from build123d import *

# Parameters (mm, degrees)
SKETCH1_W           = 35
SKETCH1_H           = 35
BOSS_EXTRUDE1_DEPTH = 9.6
SKETCH2_R           = 10
SKETCH2_R_2         = 8
CUT_EXTRUDE1_DEPTH  = 7.6
CUT_EXTRUDE2_DEPTH  = 2
CHAMFER1_SIZE       = 2.5
SKETCH4_R           = 1.65
SKETCH4_R_2         = 2.25
CUT_EXTRUDE3_DEPTH  = 26.889380062
SKETCH5_R           = 3
CUT_EXTRUDE4_DEPTH  = 2.5
BOSS_EXTRUDE3_DEPTH = 1.25


with BuildPart() as part:
    # Sketch1 → Boss-Extrude1 (new body)
    with BuildSketch(Plane(origin=(0, 0, 0), x_dir=(1, 0, 0), z_dir=(0, 1, 0))):
        Rectangle(SKETCH1_W, SKETCH1_H)
    extrude(amount=BOSS_EXTRUDE1_DEPTH)

    # Sketch2 → Cut-Extrude1 (cut)
    # profile 1 of 2: a face of its own
    with BuildSketch(Plane(origin=(0, 9.6, 0), x_dir=(1, 0, 0), z_dir=(0, 1, 0))):
        Polygon((16.25, 7), (7, 16.25), (-7, 16.25), (-16.25, 7), (-16.25, -7), (-7, -16.25), (-4, -16.25), (-4, -17.5), (4, -17.5), (4, -16.25), (7, -16.25), (16.25, -7), align=None)
        with Locations(Location((0, 0, 0), (0, 0, 270))):
            Circle(SKETCH2_R, mode=Mode.SUBTRACT)
    # profile 2 of 2: a face of its own
    with BuildSketch(Plane(origin=(0, 9.6, 0), x_dir=(1, 0, 0), z_dir=(0, 1, 0))):
        with Locations(Location((0, 0, 0), (0, 0, 270))):
            Circle(SKETCH2_R_2)
    extrude(amount=-CUT_EXTRUDE1_DEPTH, mode=Mode.SUBTRACT)

    # Sketch3 → Cut-Extrude2 (cut)
    with BuildSketch(Plane(origin=(0, 9.6, 0), x_dir=(1, 0, 0), z_dir=(0, 1, 0))):
        Polygon((11.75, 17.5), (-11.75, 17.5), (-17.5, 11.75), (-17.5, -11.75), (-11.75, -17.5), (11.75, -17.5), (17.5, -11.75), (17.5, 11.75), align=None)
    extrude(amount=-CUT_EXTRUDE2_DEPTH, mode=Mode.SUBTRACT)

    # Chamfer1
    chamfer1_edges = [part.edges().sort_by_distance(p)[0] for p in [
        (17.5, 4.8, 17.5),
        (-17.5, 4.8, 17.5),
        (-17.5, 4.8, -17.5),
        (17.5, 4.8, -17.5),
    ]]
    chamfer(chamfer1_edges, length=CHAMFER1_SIZE)

    # Sketch4 → Cut-Extrude3 (cut, through all)
    with BuildSketch(Plane(origin=(0, 7.6, 0), x_dir=(1, 0, 0), z_dir=(0, 1, 0))):
        with Locations(Location((-13, 13, 0), (0, 0, 270))):
            Circle(SKETCH4_R)
        with Locations(Location((13, 13, 0), (0, 0, 90))):
            Circle(SKETCH4_R)
        with Locations(Location((13, -13, 0), (0, 0, 270))):
            Circle(SKETCH4_R)
        with Locations(Location((-13, -13, 0), (0, 0, 90))):
            Circle(SKETCH4_R)
        with Locations(Location((0, 0, 0), (0, 0, 270))):
            Circle(SKETCH4_R_2)
    extrude(amount=-CUT_EXTRUDE3_DEPTH, mode=Mode.SUBTRACT)

    # Sketch5 → Cut-Extrude4 (cut)
    with BuildSketch(Plane.XZ):
        with Locations(Location((13, 13, 0), (0, 0, 270))):
            Circle(SKETCH5_R)
        with Locations(Location((13, -13, 0), (0, 0, 184.59538669))):
            Circle(SKETCH5_R)
        with Locations(Location((-13, -13, 0), (0, 0, 270))):
            Circle(SKETCH5_R)
        with Locations(Location((-13, 13, 0), (0, 0, 265.40461331))):
            Circle(SKETCH5_R)
    extrude(amount=-CUT_EXTRUDE4_DEPTH, mode=Mode.SUBTRACT)

    # Sketch6 → Boss-Extrude3 (add)
    with BuildSketch(Plane(origin=(0, 2, 0), x_dir=(1, 0, 0), z_dir=(0, 1, 0))):
        Polygon((13.392766953, 9.857233047), (9.857233047, 13.392766953), (8.973349571, 12.508883476), (12.508883476, 8.973349571), align=None)
        Polygon((9.857233047, -13.392766953), (8.973349571, -12.508883476), (12.508883476, -8.973349571), (13.392766953, -9.857233047), align=None)
        Polygon((-13.392766953, -9.857233047), (-9.857233047, -13.392766953), (-8.973349571, -12.508883476), (-12.508883476, -8.973349571), align=None)
        Polygon((-9.857233047, 13.392766953), (-8.973349571, 12.508883476), (-12.508883476, 8.973349571), (-13.392766953, 9.857233047), align=None)
    extrude(amount=BOSS_EXTRUDE3_DEPTH)


solid = part.part
Verification items for the finished model (mm, model axes). A direction names the side the tool comes from. Coordinates: 2 decimals unless noted, no trailing zeros. Order: outer loops, then holes, each group sorted by start corner. A loop starts at its lowest first (then second) coordinate and runs counter-clockwise, first axis right, second up. Notation, with made-up numbers: (67.25, 77.5) -> (85.25, 77.5) arc R25 ccw to (85.25, 95.5) -> close; hole circle Ø3 at (-9.75, -12). An arc over 180 degrees is marked (long way). Put each result on its own line as item: value. Start each with the question number.
1. Go/stop test with flat-tipped pins: pin 1 Ø4.5 at (x, y) = (-2, 5) entering from +Z; pin 2 Ø3.5 at (x, z) = (11.5, -10.5) entering from +Y; pin 3 Ø1.8 at (x, z) = (-12, -12) entering from -Y; pin 4 Ø1.8 at (x, z) = (-14.5, 14) entering from -Y. Record where each tip stops, or that it passes through.
2. Cross-section at C-C, the plane z = 0. Record the boundary of the cut face in (x, y), then the cut area to 3 significant figures.
3. Cross-section at D-D, the plane y = 9. Record the boundary of the cut face in (x, z), then the cut area to 3 significant figures.
4. Mould release check, pull along X, two halves, no side actions. Record for faces 4 (the cylindrical face through (-15.662, 1.232, -14.384)), 5 (the flat face through (15, 9.6, 15)), 6 (the flat face through (-14.3, 2.5, -14.3)): released by +X, released by -X, zero draft, split by the parting line, or undercut.
5. Material ranges on L1, parallel to Z at x = 13, y = 0.7; L2, parallel to Z at x = -6, y = 7.25; L3, parallel to X at y = 5.3, z = 0, recorded low to high. Write a range as [from, to].
6. Access from +Z, -Z, +X, -X, +Y, -Y to the whole of each face (thin tool, end or side, straight path). Record for faces 1 (the flat face through (-14.2, 2.5, 14.5)), 2 (the flat face through (10.716, 2.616, 10.766)), 3 (the flat face through (-4, 5, 17)).
7. Cross-section at A-A, the plane y = 5. Record the boundary of the cut face in (x, z), then the cut area to 3 significant figures.
8. Cross-section at B-B, the plane x = 0. Record the boundary of the cut face in (y, z).
Computed:
1. pin 1: z = 17.5
1. pin 2: y = 7.6
1. pin 3: y = 2
1. pin 4: y = 2.5
2. outline: (-17.5, 0) -> (-2.25, 0) -> (-2.25, 2) -> (-8, 2) -> (-8, 7.6) -> (-10, 7.6) -> (-10, 2) -> (-16.25, 2) -> (-16.25, 7.6) -> (-17.5, 7.6) -> close; (2.25, 0) -> (17.5, 0) -> (17.5, 7.6) -> (16.25, 7.6) -> (16.25, 2) -> (10, 2) -> (10, 7.6) -> (8, 7.6) -> (8, 2) -> (2.25, 2) -> close
2. area: 97.4 mm2
3. outline: (-17.5, -15) -> (-15, -17.5) -> (-11.75, -17.5) -> (-17.5, -11.75) -> close; (-17.5, 11.75) -> (-11.75, 17.5) -> (-15, 17.5) -> (-17.5, 15) -> close; (11.75, -17.5) -> (15, -17.5) -> (17.5, -15) -> (17.5, -11.75) -> close; (11.75, 17.5) -> (17.5, 11.75) -> (17.5, 15) -> (15, 17.5) -> close
3. area: 53.6 mm2
4. face 4: undercut
4. face 5: zero draft
4. face 6: undercut
5. L1: [-17.5, -16], [-10, 10], [16, 17.5]
5. L2: [-17.5, -16.25], [-8, -5.29], [5.29, 8], [16.25, 17.5]
5. L3: [-17.5, -16.25], [-10, -8], [8, 10], [16.25, 17.5]
6. face 1: -Y
6. face 2: +Y
6. face 3: +Z, +Y
7. outline: (-17.5, -15) -> (-15, -17.5) -> (15, -17.5) -> (17.5, -15) -> (17.5, 15) -> (15, 17.5) -> (4, 17.5) -> (4, 16.25) -> (7, 16.25) -> (16.25, 7) -> (16.25, -7) -> (7, -16.25) -> (-7, -16.25) -> (-16.25, -7) -> (-16.25, 7) -> (-7, 16.25) -> (-4, 16.25) -> (-4, 17.5) -> (-15, 17.5) -> (-17.5, 15) -> close; circle Ø20 at (0, 0); hole circle Ø3.3 at (-13, -13); hole circle Ø3.3 at (-13, 13); hole circle Ø16 at (0, 0); hole circle Ø3.3 at (13, -13); hole circle Ø3.3 at (13, 13)
7. area: 396 mm2
8. outline: (0, -17.5) -> (7.6, -17.5) -> (7.6, -16.25) -> (2, -16.25) -> (2, -10) -> (7.6, -10) -> (7.6, -8) -> (2, -8) -> (2, -2.25) -> (0, -2.25) -> close; (0, 2.25) -> (2, 2.25) -> (2, 8) -> (7.6, 8) -> (7.6, 10) -> (2, 10) -> (2, 17.5) -> (0, 17.5) -> close
